Autodesk Inventor part; units mm, degrees
ref_plane "Work Plane1" through (0, 0.3937, 0) normal (0, 1, 0) x (1, 0, 0)
ref_plane "YZ Plane" through (0, 0, 0) normal (1, 0, 0) x (0, 1, 0)
ref_plane "XZ Plane" through (0, 0, 0) normal (0, 1, 0) x (-1, 0, 0)
sketch "Sketch1" plane through (0, 0, 0) normal (0, 0, 1) x (1, 0, 0)
  line L0 (0, 0) -> (0, 38.608)
  line L1 (0, 38.608) -> (3.9116, 38.608)
  line L2 (3.9116, 38.608) -> (3.9116, 5.1562)
  line L3 (3.9116, 5.1562) -> (6.731, 5.1562)
  line L4 (6.731, 5.1562) -> (3.9116, 5.1562)
  line L5 (6.731, 5.1562) -> (3.9116, 5.1562)
  arc A0 (0, 0) -> (6.731, 5.1562) centre (0, 6.9715) ccw
  dimension "d0" = 38.608
  dimension "d1" = 6.731
  dimension "d3" = 3.9116
  dimension "d4" = 33.4518
revolve "Revolution1" add sketch "Sketch1" angle 360 about axis through (0, 0, 0) along (0, 1, 0)
fillet "Fillet1" radius 0.3175 1 edges at (-6.731, 5.1562, 0)
sketch "Sketch2" plane through (0, 5.1562, 0) normal (0, 1, 0) x (1, 0, 0)
  point P0 (0, 0)
ref_plane "Work Plane1" through (0, 0.3937, 0) normal (0, 1, 0) x (1, 0, 0)
sketch "Sketch3" plane through (0, 0.3937, 0) normal (0, 1, 0) x (1, 0, 0)
  line L0 (0, 2.8575) -> (2.4747, 1.4287)
  line L1 (2.4747, 1.4287) -> (2.4747, -1.4287)
  line L2 (2.4747, -1.4287) -> (0, -2.8575)
  line L3 (0, -2.8575) -> (-2.4747, -1.4288)
  line L4 (-2.4747, -1.4288) -> (-2.4747, 1.4287)
  line L5 (-2.4747, 1.4287) -> (0, 2.8575)
  point P0 (0, 0)
  point P1 (0, 0)
  dimension "d9" = 5.715
extrude "Extrusion1" cut sketch "Sketch3" along normal blind 4.572 and the other way blind 2.286
fillet "Fillet2" radius 0.3175 1 edges at (-3.9116, 5.1562, 0)
fillet "Fillet3" radius 0.3175 1 edges at (-3.9116, 38.608, 0)
sketch "Sketch4" plane through (0, 38.608, 0) normal (0, 1, 0) x (1, 0, 0)
  circle A0 centre (0, 0) radius 3.5941
  circle A1 centre (0, 0) radius 2.6035
  dimension "d16" = 5.207
extrude "Extrusion2" cut sketch "Sketch4" against normal blind 19.558 contours A1
thread "Thread1"
properties part number "Axel-Female" material "Stainless Steel"
Geometry check sheet. Reference: the model listing, model coordinates, mm. A direction names the side the tool comes from. Coordinates: 2 decimals unless noted, no trailing zeros. Write each loop counter-clockwise with the first axis right and the second up, starting at its lowest first coordinate (ties: lowest second). Pieces come first, ordered by that corner, then holes. Notation, with made-up numbers: M 42.25,76.25 L 76.25,76.25 A5 ccw 76.25,80.25 Z; hole C 1.25,13 d7. An arc over 180 degrees is marked long. Answer as a JSON object with one key per item and string values.
1. Section check A-A, the plane y = 11. Enter the section's corners in (x, z), plus the area to 3 significant figures.
Answers below:
{"outline": "C 0,0 d7.82", "area": "48.1 mm²"}
2. Go/stop test with flat-tipped pins: pin 1 Ø6 at (x, y) = (4, 27) entering from +Z; pin 2 Ø3 at (y, z) = (3, 0.5) entering from +X; pin 3 Ø2.5 at (y, z) = (3.5, -0.5) entering from -X; pin 4 Ø1 at (x, y) = (-5, 13) entering from -Z. Record where each tip stops, or that it passes through.
Answers below:
{"pin 1": "stops at z = 3.78", "pin 2": "stops at x = 6.51", "pin 3": "stops at x = -6.6", "pin 4": "passes through"}
3. Draft check along Z on faces 4 (the flat face through (1.255, 2.678, 2.133)), 5 (the flat face through (-4, 5.156, 2)), 6 (the cylindrical face through (3.731, 21.652, 1.175)). Enter one of: released by +Z, released by -Z, zero draft, split by the parting line, or undercut.
Answers below:
{"face 4": "undercut", "face 5": "zero draft", "face 6": "split by the parting line"}
4. Section check B-B, the plane y = 20.5. Enter the section's corners in (x, z).
Answers below:
{"outline": "C 0,0 d7.82; hole C 0,0 d5.21"}
5. Tool access check on faces 1 (the flat face through (-2.475, 3, 0)), 2 (the flat face through (0, 19.05, 0)), 3 (the flat face through (2, 38.608, -2)). Record the directions out of +Z, -Z, +X, -X, +Y, -Y that give a thin tool (end or side, any length) a straight path to the whole face; none if there is none.
Answers below:
{"face 1": "-Y", "face 2": "+Y", "face 3": "+Z, -Z, +X, -X, +Y"}
6. Scan lines: L1, parallel to X at y = 33.25, z = 0; L2, parallel to Z at x = -1.25, y = 22. Record each from-to range of solid material in increasing order.
Answers below:
{"L1": "x = -3.91 to -2.6, 2.6 to 3.91", "L2": "z = -3.71 to -2.28, 2.28 to 3.71"}
